Design review of the part built by this model. Coordinates are the model's own, in mm. Face numbers are marked on the shaded views. Coordinates: 2 decimals unless noted, no trailing zeros. Write each loop counter-clockwise with the first axis right and the second up, starting at its lowest first coordinate (ties: lowest second). Pieces come first, ordered by that corner, then holes. Notation, with made-up numbers: (73, 9) -> (118, 9) arc R30 ccw to (118, 39) -> close; hole circle Ø11 at (42.5, 27.5). An arc over 180 degrees is marked (long way). Answer in a Markdown table with one row per item. Add a question column.
Item 1: Clearance check with flat-ended pins moving along their axes: P1, Ø0.6, axis at y = 11, z = 7.5, coming from the -X side; P2, Ø1.5, axis at x = 4.5, y = 11, coming from the +Z side; P3, Ø6, axis at x = -1.5, z = -2, coming from the +Y side. State where each tip first meets the part, or that it passes through.
Item 2: Draft analysis for pull direction Z (two halves, no side actions). For the marked faces 1, 2, 3 and 4, state which applies: released by +Z, released by -Z, zero draft, split by the parting line, or undercut.
Item 3: To check wall thickness, follow line 1 (X direction, y = 14.5, z = 0); line 2 (Y direction, x = 5.25, z = -0.75); line 3 (X direction, y = 21.75, z = -5.25). State the ranges of each line that lie inside material, in increasing order.
Item 4: Take a section at A-A, the plane y = 19.5. Write out the cut boundary in (x, z), and give its area (3 significant figures).
Item 5: Take a section at B-B, the plane x = -0.75. Write out the cut boundary in (y, z), and give its area (3 significant figures).
Item 6: Take a section at C-C, the plane z = -0.5. Write out the cut boundary in (x, y), and give its area (3 significant figures).
Item 7: Take a section at D-D, the plane y = 10.5. Write out the cut boundary in (x, z), and give its area (3 significant figures).
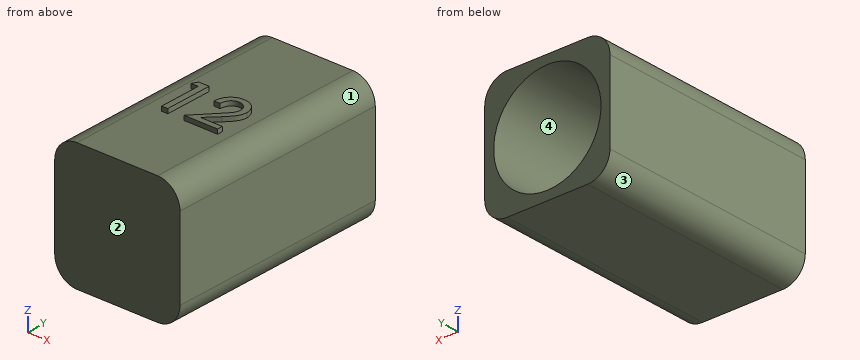
from build123d import *

# Parameters (mm, degrees)
SKETCH1_W           = 14
SKETCH1_H           = 14
BOSS_EXTRUDE1_DEPTH = 25
SKETCH2_R           = 6
CUT_EXTRUDE1_DEPTH  = 24
BOSS_EXTRUDE3_DEPTH = 0.5
FILLET1_R           = 2.5
FILLET2_R           = 2.5
FILLET3_R           = 2.5
FILLET4_R           = 2.5


with BuildPart() as part:
    # Sketch1 → Boss-Extrude1 (new body)
    with BuildSketch(Plane(origin=(0, 0, 0), x_dir=(1, 0, 0), z_dir=(0, 1, 0))):
        Rectangle(SKETCH1_W, SKETCH1_H)
    extrude(amount=BOSS_EXTRUDE1_DEPTH)

    # Sketch2 → Cut-Extrude1 (cut)
    with BuildSketch(Plane(origin=(0, 25, 0), x_dir=(1, 0, 0), z_dir=(0, 1, 0))):
        with Locations(Location((0, 0, 0), (0, 0, 270))):
            Circle(SKETCH2_R)
    extrude(amount=-CUT_EXTRUDE1_DEPTH, mode=Mode.SUBTRACT)

    # Sketch3 → Boss-Extrude3 (add)
    with BuildSketch(Plane.XY.offset(7)):
        Polygon((-3.300679086, 14.210073329), (-2.149487179, 14.210073329), (-2.149487179, 8.918406662), (-2.827905982, 8.918406662), (-2.827905982, 13.599496406), (-3.642008546, 13.599496406), align=None)
        with BuildLine():
            Line((0.556767829, 12.514026321), (-0.114230768, 12.514026321))
            add(Edge.make_bspline(
                [(-0.114230768, 12.514026321), (-0.111078886, 12.582304036), (-0.104914236, 12.71584588), (-0.077540014, 12.910431266), (-0.033195725, 13.093780337), (0.02277613, 13.267447402), (0.097441024, 13.429261532), (0.183589376, 13.582043561), (0.287590231, 13.722591478), (0.405116879, 13.851127618), (0.532696206, 13.967907704), (0.66984458, 14.068604955), (0.814243771, 14.154413881), (0.965922174, 14.224434532), (1.125176835, 14.278650186), (1.291553818, 14.318101559), (1.465583884, 14.341830622), (1.584215771, 14.344436169), (1.644357974, 14.34575709)],
                knots=[0, 0, 0, 0, 1.154964179, 2.258951466, 3.315045469, 4.34063582, 5.337653555, 6.322213479, 7.300594401, 8.285733883, 9.262436119, 10.219305053, 11.156568068, 12.097250375, 13.037875795, 13.995471444, 14.983774372, 16, 16, 16, 16], degree=3))
            add(Edge.make_bspline(
                [(1.644357974, 14.34575709), (1.70732699, 14.344469016), (1.830889612, 14.34194146), (2.01082655, 14.31815685), (2.181120391, 14.279804182), (2.341820997, 14.227428226), (2.492635583, 14.157492683), (2.633861547, 14.073158132), (2.764141354, 13.971791047), (2.884420569, 13.858367608), (2.990658217, 13.73360089), (3.086612633, 13.605325884), (3.165928247, 13.470941026), (3.232374739, 13.332900213), (3.283506362, 13.190070488), (3.319615354, 13.043033103), (3.341259687, 12.891688146), (3.344213908, 12.789350264), (3.345705129, 12.73769252)],
                knots=[0, 0, 0, 0, 1.156722346, 2.269809107, 3.328396062, 4.361258308, 5.3694338, 6.377253737, 7.377324894, 8.397019439, 9.4098266, 10.385180797, 11.337325354, 12.27255833, 13.196816462, 14.119704983, 15.050871513, 16, 16, 16, 16], degree=3))
            add(Edge.make_bspline(
                [(3.345705129, 12.73769252), (3.342991558, 12.665431813), (3.337601589, 12.521900312), (3.29609716, 12.309553694), (3.226323351, 12.104046507), (3.145727927, 11.936709759), (3.064215379, 11.80144908), (2.989411872, 11.689803537), (2.901537104, 11.569080813), (2.798706557, 11.440089036), (2.685009192, 11.299876822), (2.555928501, 11.152061213), (2.415459729, 10.993649578), (2.315279585, 10.886982507), (2.263415132, 10.831759694)],
                knots=[0, 0, 0, 0, 1.155755081, 2.295677249, 3.447123235, 4.6205014, 5.259503175, 5.973005395, 6.77029923, 7.648035671, 8.612336498, 9.658570495, 10.787814065, 12, 12, 12, 12], degree=3))
            Line((2.263415132, 10.831759694), (0.961699053, 9.528983586))
            Line((0.961699053, 9.528983586), (3.413547009, 9.528983586))
            Line((3.413547009, 9.528983586), (3.413547009, 8.918406662))
            Line((3.413547009, 8.918406662), (-0.317756409, 8.918406662))
            Line((-0.317756409, 8.918406662), (1.706899707, 11.154008626))
            add(Edge.make_bspline(
                [(1.706899707, 11.154008626), (1.755124332, 11.205439648), (1.847668268, 11.304136719), (1.978095845, 11.448613384), (2.095770717, 11.582179805), (2.201320257, 11.704739563), (2.29198055, 11.81793999), (2.370190541, 11.92011571), (2.435064878, 12.011749217), (2.502437185, 12.119609483), (2.569196231, 12.248904612), (2.625986943, 12.406626513), (2.660064153, 12.567694788), (2.664877757, 12.676053287), (2.667286326, 12.730272314)],
                knots=[0, 0, 0, 0, 1.341560447, 2.574479018, 3.703506985, 4.728875774, 5.651874962, 6.462761537, 7.177175968, 7.787249671, 8.88179658, 9.938774664, 10.968630673, 12, 12, 12, 12], degree=3))
            add(Edge.make_bspline(
                [(2.667286326, 12.730272314), (2.666692753, 12.763907746), (2.66551825, 12.830462259), (2.649505827, 12.927923363), (2.626949455, 13.022455211), (2.592062636, 13.112538015), (2.550030438, 13.199944057), (2.497455636, 13.283543423), (2.434322648, 13.362560638), (2.36409314, 13.43877354), (2.286417458, 13.507585159), (2.204373375, 13.569299116), (2.116951948, 13.619418877), (2.026543408, 13.663249485), (1.930337353, 13.694322519), (1.830698643, 13.717457991), (1.726844914, 13.733484398), (1.656080047, 13.734607291), (1.619977298, 13.735180167)],
                knots=[0, 0, 0, 0, 0.999432927, 1.977580462, 2.931018689, 3.885672852, 4.844657058, 5.812871023, 6.815890212, 7.849665183, 8.891901864, 9.898878619, 10.897592748, 11.885014695, 12.882178885, 13.896915602, 14.927050508, 16, 16, 16, 16], degree=3))
            add(Edge.make_bspline(
                [(1.619977298, 13.735180167), (1.585654597, 13.734476202), (1.518132832, 13.733091317), (1.41869032, 13.718802518), (1.32323782, 13.695537542), (1.23145333, 13.663266899), (1.14267207, 13.623454267), (1.059064891, 13.571877079), (0.979265259, 13.511876917), (0.902218203, 13.444535768), (0.832096498, 13.365531193), (0.76937784, 13.275799414), (0.71399479, 13.175242657), (0.666655887, 13.064036834), (0.627423824, 12.941890194), (0.595952005, 12.808951264), (0.571621246, 12.66516219), (0.561810561, 12.565336908), (0.556767829, 12.514026321)],
                knots=[0, 0, 0, 0, 0.911540883, 1.79324023, 2.663162255, 3.518366492, 4.375475705, 5.243419306, 6.122264358, 7.02676621, 7.957780629, 8.921596253, 9.930241338, 11.002848587, 12.128200329, 13.335197372, 14.630280975, 16, 16, 16, 16], degree=3))
        make_face()
    extrude(amount=BOSS_EXTRUDE3_DEPTH)

    # Fillet1
    fillet1_edges = [part.edges().sort_by_distance(p)[0] for p in [
        (-7, 12.5, 7),
    ]]
    fillet(fillet1_edges, radius=FILLET1_R)

    # Fillet2
    fillet2_edges = [part.edges().sort_by_distance(p)[0] for p in [
        (7, 12.5, 7),
    ]]
    fillet(fillet2_edges, radius=FILLET2_R)

    # Fillet3
    fillet3_edges = [part.edges().sort_by_distance(p)[0] for p in [
        (7, 12.5, -7),
    ]]
    fillet(fillet3_edges, radius=FILLET3_R)

    # Fillet4
    fillet4_edges = [part.edges().sort_by_distance(p)[0] for p in [
        (-7, 12.5, -7),
    ]]
    fillet(fillet4_edges, radius=FILLET4_R)


solid = part.part
Answers:
| question | item | result |
|---|---|---|
| 1 | P1 | stops at x = -2.83 |
| 1 | P2 | stops at z = 7 |
| 1 | P3 | stops at y = 1 |
| 2 | face 1 | released by +Z |
| 2 | face 2 | zero draft |
| 2 | face 3 | released by -Z |
| 2 | face 4 | undercut |
| 3 | line 1 | x = -7 to -6, 6 to 7 |
| 3 | line 2 | y = 0 to 1 |
| 3 | line 3 | x = -6.88 to -2.9, 2.9 to 6.88 |
| 4 | outline | (-7, -4.5) arc R2.5 ccw to (-4.5, -7) -> (4.5, -7) arc R2.5 ccw to (7, -4.5) -> (7, 4.5) arc R2.5 ccw to (4.5, 7) -> (-4.5, 7) arc R2.5 ccw to (-7, 4.5) -> close; hole circle Ø12 at (0, 0) |
| 4 | area | 77.5 mm^2 |
| 5 | outline | (0, -7) -> (25, -7) -> (25, -5.95) -> (1, -5.95) -> (1, 5.95) -> (25, 5.95) -> (25, 7) -> (0, 7) -> close |
| 5 | area | 64.3 mm^2 |
| 6 | outline | (-7, 0) -> (7, 0) -> (7, 25) -> (5.98, 25) -> (5.98, 1) -> (-5.98, 1) -> (-5.98, 25) -> (-7, 25) -> close |
| 6 | area | 63.0 mm^2 |
| 7 | outline | (-7, -4.5) arc R2.5 ccw to (-4.5, -7) -> (4.5, -7) arc R2.5 ccw to (7, -4.5) -> (7, 4.5) arc R2.5 ccw to (4.5, 7) -> (1.93, 7) -> (1.93, 7.5) -> (1.11, 7.5) -> (1.11, 7) -> (-2.15, 7) -> (-2.15, 7.5) -> (-2.83, 7.5) -> (-2.83, 7) -> (-4.5, 7) arc R2.5 ccw to (-7, 4.5) -> close; hole circle Ø12 at (0, 0) |
| 7 | area | 78.3 mm^2 |
